Source: three-view drawing plus pictorial views. Frame: mm from the lowest corner of the part. A direction names the side the tool comes from. Give positions to 0.01 mm unless a question says otherwise; leave off trailing zeros. Loops run counter-clockwise (first coordinate to the right, second up) from the corner with the lowest first, then second, coordinate; pieces in that order, holes last. Notation, with made-up numbers: M 19.5,59.25 L 74.5,59.25 A9 cw 74.5,63.25 Z; hole C -22,83 d11. An arc over 180 degrees is marked long. One line per item, written item: value. Start each with the question number.
(1) Section D-D on z = 41. Output: boundary loops of the cut face in (x, y).
(2) Section A-A on x = 40. Output: boundary loops of the cut face in (y, z).
(3) Ray query, line 1 along X through (y, z) = (6.7, 6); line 2 along Z through (x, y) = (40, 3.5); line 3 along Z through (x, y) = (22.5, 8). Return the intervals inside material, ascending. Write a range as from..to.
(4) Section C-C on y = 3.5. Output: boundary loops of the cut face in (x, z), plus the area to 3 significant figures.
(5) Section B-B on z = 61. Output: boundary loops of the cut face in (x, y), plus the area to 3 significant figures.
(6) Pull-direction query (Z, two-part tool) for the marked faces 1, 2 and 3; classes: released by +Z, released by -Z, zero draft, split by the parting line, or undercut.
(7) Pin query (flat end, axial travel): P1, Ø6, axis at x = 23, z = 37.5, coming from the +Y side; P2, Ø1.5, axis at x = 5.5, y = 5.5, coming from the -Z side; P3, Ø1.8, axis at x = 40, z = 58.5, coming from the +Y side. Return the tip coordinate at first contact, or that it passes through.
(8) Access query for the marked faces 4 and 5. Directions: +Z, -Z, +X, -X, +Y, -Y. A direction counts if a zero-diameter tool reaches every point of the face in a straight line with its end or side. Return the directions, or none.
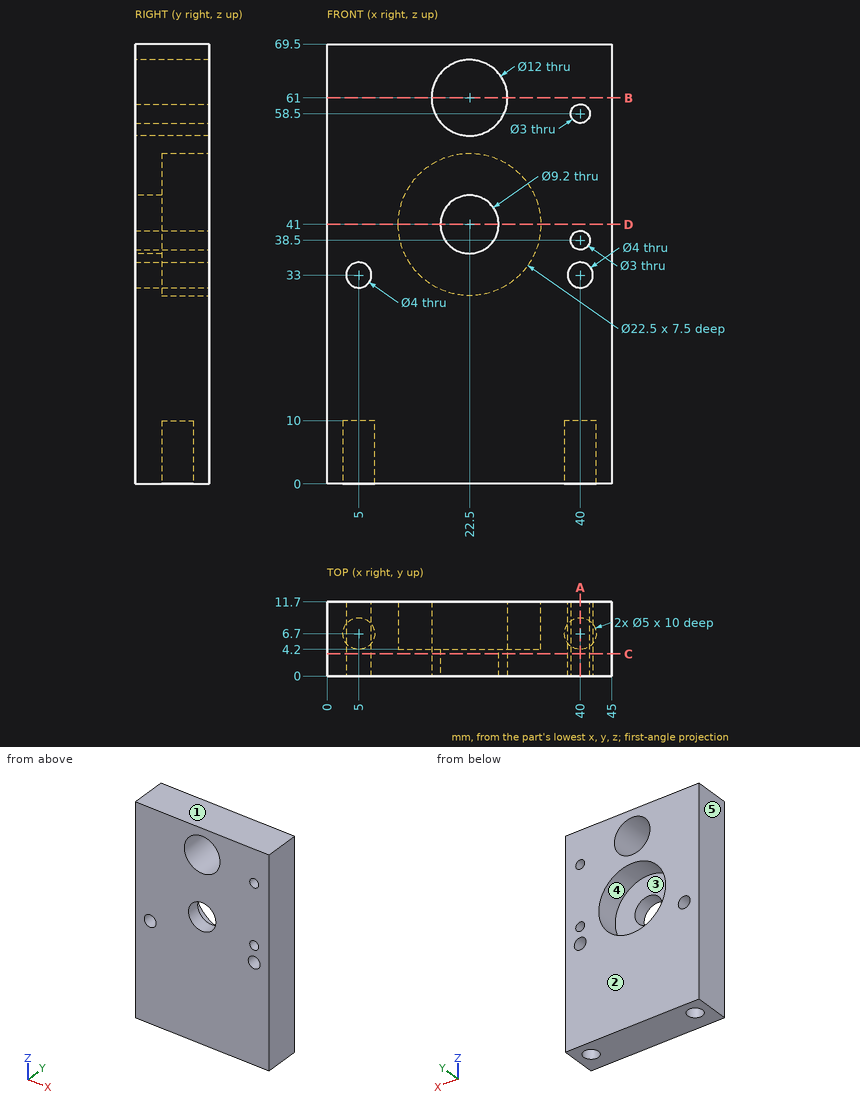
Output values:
1. outline: M 0,0 L 17.9,0 L 17.9,4.2 L 11.25,4.2 L 11.25,11.7 L 0,11.7 Z; M 27.1,0 L 45,0 L 45,11.7 L 33.75,11.7 L 33.75,4.2 L 27.1,4.2 Z
2. outline: M 0,0 L 4.2,0 L 4.2,10 L 9.2,10 L 9.2,0 L 11.7,0 L 11.7,31 L 0,31 Z; M 0,35 L 11.7,35 L 11.7,37 L 0,37 Z; M 0,40 L 11.7,40 L 11.7,57 L 0,57 Z; M 0,60 L 11.7,60 L 11.7,69.5 L 0,69.5 Z
3. line 1: x = 0..2.5, 7.5..37.5, 42.5..45
3. line 2: z = 0..31, 35..37, 40..57, 60..69.5
3. line 3: z = 0..29.75, 52.25..55, 67..69.5
4. outline: M 0,0 L 45,0 L 45,69.5 L 0,69.5 Z; hole C 5,33 d4; hole C 22.5,61 d12; hole C 22.5,41 d9.2; hole C 40,33 d4; hole C 40,38.5 d3; hole C 40,58.5 d3
4. area: 2,910 mm²
5. outline: M 0,0 L 16.5,0 L 16.5,11.7 L 0,11.7 Z; M 28.5,0 L 45,0 L 45,11.7 L 28.5,11.7 Z
5. area: 386 mm²
6. face 1: released by +Z
6. face 2: zero draft
6. face 3: undercut
7. P1: stops at y = 4.2
7. P2: stops at z = 10
7. P3: passes through
8. face 4: +Y
8. face 5: +Z, -Z, -X, +Y, -Y
